Input: dimensioned drawing with shaded views. Units: mm. Origin: part minimum x, y, z. A direction names the side the tool comes from. Round coordinates to 2 decimals unless told otherwise and drop trailing zeros. Order: outer loops, then holes, each group sorted by start corner. A loop starts at its lowest first (then second) coordinate and runs counter-clockwise, first axis right, second up.
Item 1: Mould query, pull axis X, two halves, no side actions, for the marked faces 1, 2 and 3. Classes: released by +X, released by -X, zero draft, split by the parting line, or undercut.
Item 2: Cut plane A-A on x = 13.2. Output: boundary loops of the cut face in (y, z), then the cut area to 3 significant figures.
Item 3: First-contact query: pin 1 (4 mm diameter, centred on x = 20.5, z = 18.5, fed in from -Y); pin 2 (6 mm diameter, centred on x = 32.2, z = 15, fed in from +Y). Flat tips, straight axial feed; report the tip coordinate or a pass-through.
Item 4: Reachability of the marked faces 4 and 5 from +Z, -Z, +X, -X, +Y, -Y: full face, straight path, thin tool, end or side. Return the list, or none.
Item 5: Cut plane B-B on z = 15. Output: boundary loops of the cut face in (x, y).
Item 6: Line query: L1, parallel to X at y = 23.65, z = 15; L2, parallel to Y at x = 6, z = 18.5; L3, parallel to X at y = 8.5, z = 28. Output: solid intervals per line, ascending.
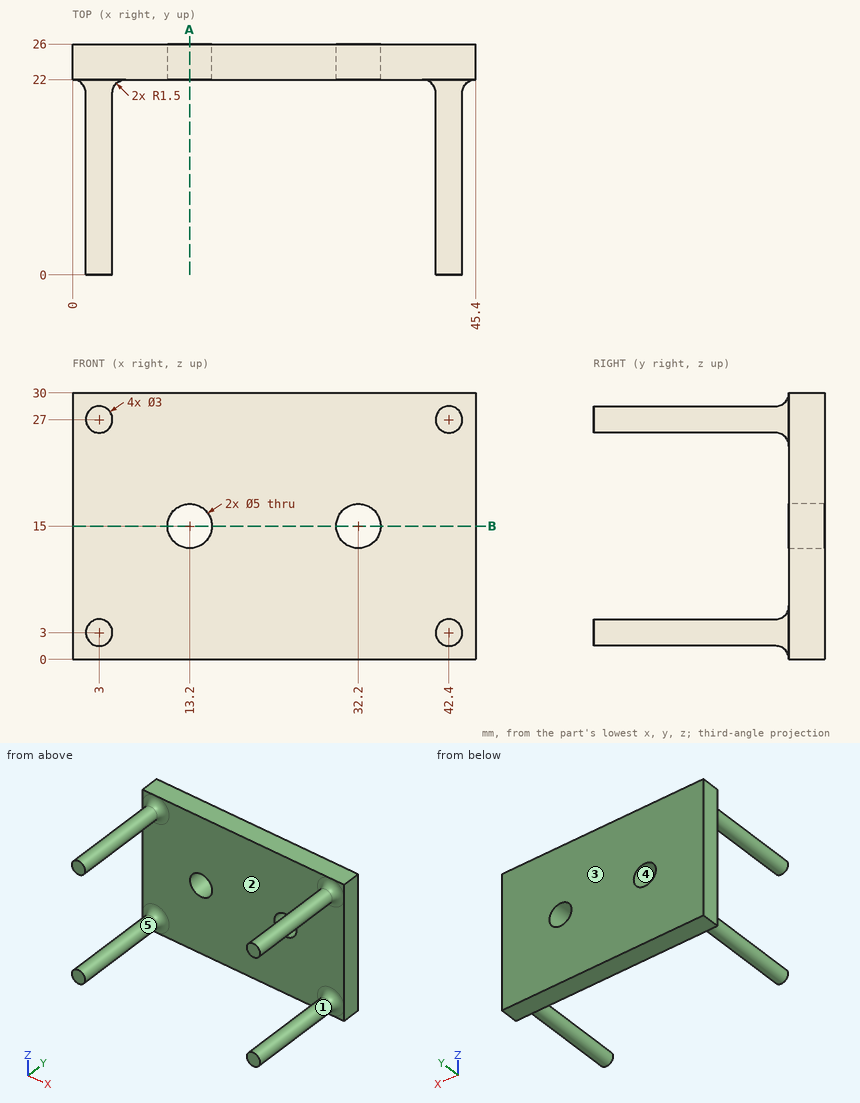
From the geometry:
1. face 1: undercut
1. face 2: undercut
1. face 3: zero draft
2. outline: (22, 0) - (26, 0) - (26, 12.5) - (22, 12.5) - close; (22, 17.5) - (26, 17.5) - (26, 30) - (22, 30) - close
2. area: 100 mm2
3. pin 1: stops at y = 22
3. pin 2: stops at y = 26
4. face 4: +Y, -Y
4. face 5: -Y
5. outline: (0, 22) - (10.7, 22) - (10.7, 26) - (0, 26) - close; (15.7, 22) - (29.7, 22) - (29.7, 26) - (15.7, 26) - close; (34.7, 22) - (45.4, 22) - (45.4, 26) - (34.7, 26) - close
6. L1: x = 0 to 10.7, 15.7 to 29.7, 34.7 to 45.4
6. L2: y = 22 to 26
6. L3: x = 1.88 to 4.12, 41.28 to 43.52
